Check sheet for the drawn part. Datum: minimum x, y, z corner. Units: mm. A direction names the side the tool comes from. Coordinates: 2 decimals unless noted, no trailing zeros. Write each loop counter-clockwise with the first axis right and the second up, starting at its lowest first coordinate (ties: lowest second). Pieces come first, ordered by that corner, then holes. Notation, with made-up numbers: (29, 17.25) - (50, 17.25) arc R14 ccw to (50, 37.25) - close; hole circle Ø9 at (69.25, 8.25). An arc over 180 degrees is marked (long way). Use CSV: the item, a comma, the result in double quotes. Start each with the question number.
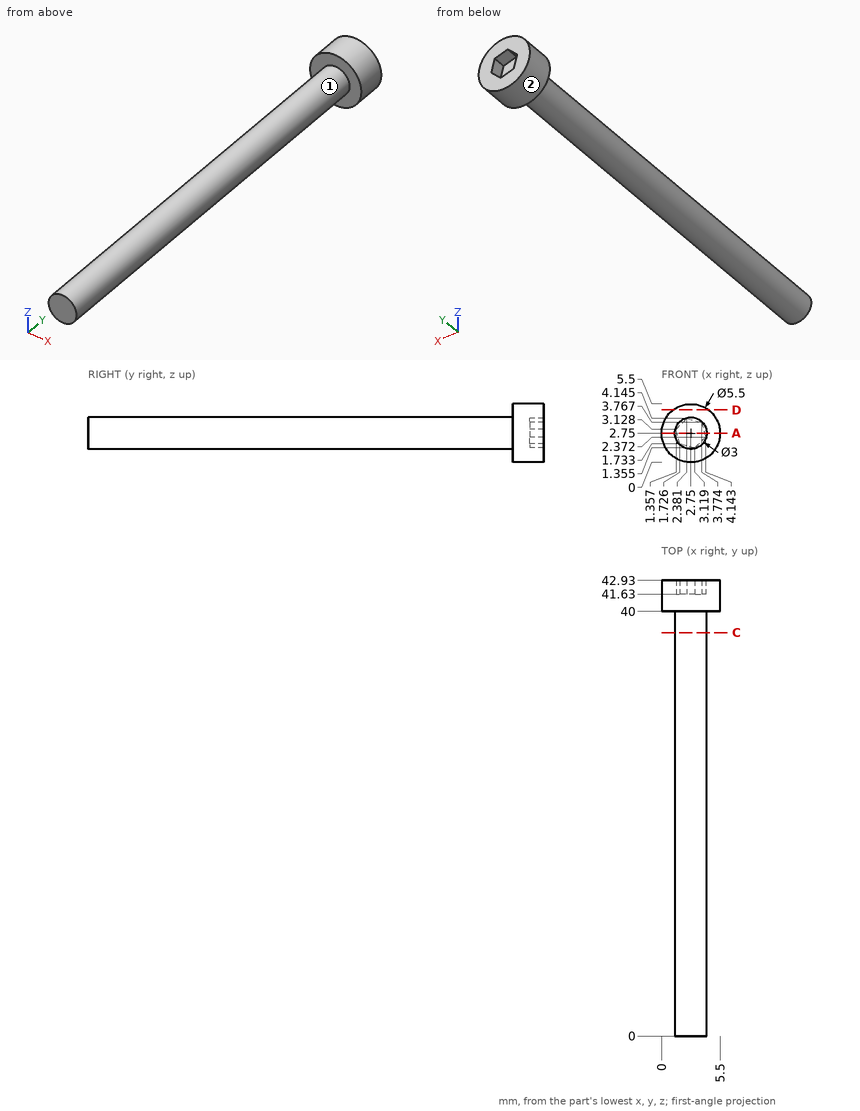
Q1. Cross-section at D-D (z = 4.95). Record the cut outline in (x, y).
Q2. Cross-section at A-A (z = 2.75). Record the cut outline in (x, y).
Q3. Cross-section at C-C (y = 38). Record the cut outline in (x, z).
Q4. Gauge pin test, flat ends, axial feed: pin 1 (2 mm diameter, centred on x = 4, y = 9, fed in from -Z); pin 2 (3 mm diameter, centred on y = 25, z = 3.5, fed in from +X); pin 3 (0.8 mm diameter, centred on x = 3.5, z = 2.5, fed in from +Y). Record the tip position at first contact, or that the pin passes through.
Q5. Scan lines: line 1 along Y through (x, z) = (3.3, 4.2); line 2 along Y through (x, z) = (2.75, 3.05); line 3 along Z through (x, y) = (3.3, 29.5) (1 decimal). Record each from-to range of solid material in increasing order. Write a range as from..to.
Q6. Tool access check on the marked faces 1 and 2. Record the directions out of +Z, -Z, +X, -X, +Y, -Y that give a thin tool (end or side, any length) a straight path to the whole face; none if there is none.
Reply:
1,outline,"(1.1, 40) - (4.4, 40) - (4.4, 42.93) - (1.1, 42.93) - close"
2,outline,"(0, 40) - (1.25, 40) - (1.25, 0) - (4.25, 0) - (4.25, 40) - (5.5, 40) - (5.5, 42.93) - (4.04, 42.93) - (4.04, 41.63) - (1.46, 41.63) - (1.46, 42.93) - (0, 42.93) - close"
3,outline,"circle Ø3 at (2.75, 2.75)"
4,pin 1,"z = 1.27"
4,pin 2,"x = 4.25"
4,pin 3,"y = 41.63"
5,line 1,"40..42.93"
5,line 2,"0..41.63"
5,line 3,"1.4..4.1"
6,face 1,"-Y"
6,face 2,"+Y, -Y"
